Check sheet for the modelled part. Datum: model origin and axes. Units: mm. Give positions to 0.01 mm unless a question says otherwise; leave off trailing zeros. Order: outer loops, then holes, each group sorted by start corner. A loop starts at its lowest first (then second) coordinate and runs counter-clockwise, first axis right, second up.
from build123d import *

# Parameters (mm, degrees)
BOSS_EXTRU_1_DEPTH = 5
ESQUISSE2_R        = 1.5
BOSS_EXTRU_2_DEPTH = 2
ESQUISSE3_R        = 15
BOSS_EXTRU_3_DEPTH = 25


with BuildPart() as part:
    # Esquisse1 → Boss.-Extru.1 (new body)
    with BuildSketch(Plane.XY):
        with BuildLine():
            ThreePointArc((-1.118033989, 1), (-1.369306394, -0.612372436), (0, -1.5))
            Line((0, -1.5), (0, 1))
            Line((0, 1), (-1.118033989, 1))
        make_face()
        with BuildLine():
            Line((0, 1), (0, -1.5))
            ThreePointArc((0, -1.5), (1.060660172, -1.060660172), (1.5, 0))
            ThreePointArc((1.5, 0), (1.401258538, 0.535233135), (1.118033989, 1))
            Line((1.118033989, 1), (0, 1))
        make_face()
    extrude(amount=BOSS_EXTRU_1_DEPTH)

    # Esquisse2 → Boss.-Extru.2 (add)
    with BuildSketch(Plane.XY.offset(5)):
        with Locations(Location((0, 0, 0), (0, 0, 138.189685104))):
            Circle(ESQUISSE2_R)
    extrude(amount=BOSS_EXTRU_2_DEPTH)

    # Esquisse3 → Boss.-Extru.3 (add)
    with BuildSketch(Plane.XY.offset(7)):
        with Locations((0, 0.131238961)):
            Circle(ESQUISSE3_R)
    extrude(amount=BOSS_EXTRU_3_DEPTH)


solid = part.part
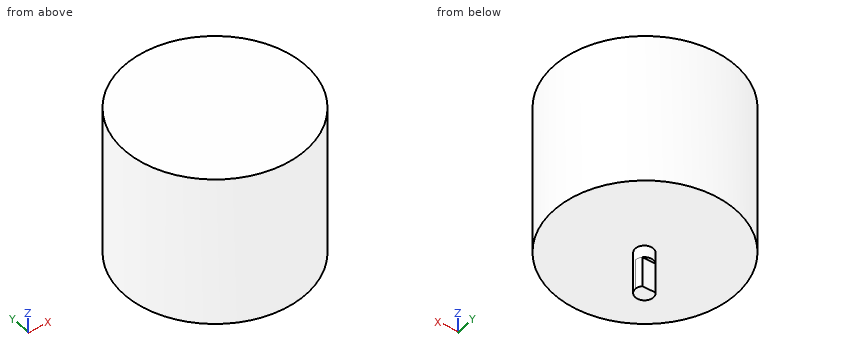
1) Section check C-C, the plane z = 17. Record the cut outline in (x, y), then the cut area to 3 significant figures.
Recorded:
outline: circle Ø30 at (0, 0.13)
area: 707 mm2
2) Section check A-A, the plane x = 0. Record the cut outline in (y, z).
Recorded:
outline: (-14.87, 7) - (-1.5, 7) - (-1.5, 0) - (1, 0) - (1, 5) - (1.5, 5) - (1.5, 7) - (15.13, 7) - (15.13, 32) - (-14.87, 32) - close
3) Depth check by flat-ended pin: pin 1 Ø9 at (x, y) = (-7.5, 2.5) entering from -Z; pin 2 Ø2.5 at (x, z) = (-0.5, 2) entering from +Y; pin 3 Ø5 at (y, z) = (10.5, 22) entering from -X; pin 4 Ø12 at (x, z) = (-2, 28.5) entering from -Y. Enter the tip coordinate at first touch or a pass-through.
Recorded:
pin 1: stops at z = 7
pin 2: stops at y = 1
pin 3: stops at x = -12.77
pin 4: stops at y = -14.87
4) Material ranges on L1, parallel to X at y = -0.25, z = 9; L2, parallel to Z at x = 13.5, y = -1; L3, parallel to Y at x = 9.25, z = 13.5, recorded low to high.
Recorded:
L1: x = -15 to 15
L2: z = 7 to 32
L3: y = -11.68 to 11.94
5) Section check B-B, the plane y = 9.25. Record the cut outline in (x, z).
Recorded:
outline: (-11.91, 7) - (11.91, 7) - (11.91, 32) - (-11.91, 32) - close
6) Section check D-D, the plane y = -9. Record the cut outline in (x, z).
Recorded:
outline: (-11.9, 7) - (11.9, 7) - (11.9, 32) - (-11.9, 32) - close
